Geometry check sheet. Reference: the model listing, model coordinates, mm. Coordinates: 2 decimals unless noted, no trailing zeros. Loops run counter-clockwise (first coordinate to the right, second up) from the corner with the lowest first, then second, coordinate; pieces in that order, holes last. Notation, with made-up numbers: (29, 58) - (46, 58) arc R14 cw to (46, 78) - close; hole circle Ø6 at (37.25, 18.25). An arc over 180 degrees is marked (long way). One line per item, written item: value.
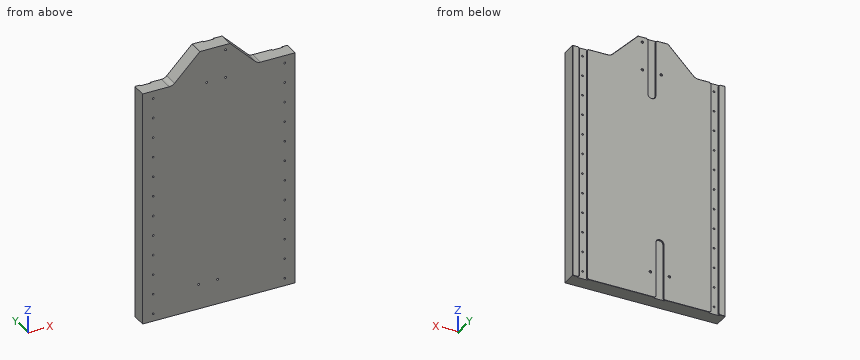
from build123d import *

# Parameters (mm, degrees)
BOSS_EXTRUDE1_DEPTH = 30
SKETCH2_R           = 1.75
SKETCH2_R_2         = 2
CUT_EXTRUDE1_DEPTH  = 31
SKETCH3_W           = 15.25
SKETCH3_H           = 470
CUT_EXTRUDE2_DEPTH  = 3
SKETCH4_W           = 15
SKETCH4_H           = 120
CUT_EXTRUDE3_DEPTH  = 3
FILLET1_R           = 7
FILLET2_R           = 15
CHAMFER1_SIZE       = 3
CHAMFER2_SIZE       = 0.5


with BuildPart() as part:
    # Sketch1 → Boss-Extrude1 (new body)
    with BuildSketch(Plane(origin=(0, 0, 0), x_dir=(1, 0, 0), z_dir=(0, 1, 0))):
        Polygon((-93, -235), (-38, -290), (22, -290), (77, -235), (152.5, -235), (152.5, 235), (-152.5, 235), (-152.5, -235), align=None)
    extrude(amount=BOSS_EXTRUDE1_DEPTH)

    # Sketch2 → Cut-Extrude1 (cut, through all)
    with BuildSketch(Plane(origin=(0, 0, 0), x_dir=(1, 0, 0), z_dir=(0, 1, 0))):
        with Locations((-131.5, 220)):
            Circle(SKETCH2_R)
        with Locations((131.5, 220)):
            Circle(SKETCH2_R)
        with Locations((13.5, -223)):
            Circle(SKETCH2_R_2)
        with Locations((-24.5, -223)):
            Circle(SKETCH2_R_2)
        with Locations((-40.5, 185)):
            Circle(SKETCH2_R_2)
        with Locations((-2.5, 185)):
            Circle(SKETCH2_R_2)
        with Locations((-131.5, 180)):
            Circle(SKETCH2_R)
        with Locations((131.5, 180)):
            Circle(SKETCH2_R)
        with Locations((-131.5, 140)):
            Circle(SKETCH2_R)
        with Locations((131.5, 140)):
            Circle(SKETCH2_R)
        with Locations((-131.5, 100)):
            Circle(SKETCH2_R)
        with Locations((131.5, 100)):
            Circle(SKETCH2_R)
        with Locations((-131.5, 60)):
            Circle(SKETCH2_R)
        with Locations((131.5, 60)):
            Circle(SKETCH2_R)
        with Locations((-131.5, 20)):
            Circle(SKETCH2_R)
        with Locations((131.5, 20)):
            Circle(SKETCH2_R)
        with Locations((-131.5, -20)):
            Circle(SKETCH2_R)
        with Locations((131.5, -20)):
            Circle(SKETCH2_R)
        with Locations((-131.5, -60)):
            Circle(SKETCH2_R)
        with Locations((131.5, -60)):
            Circle(SKETCH2_R)
        with Locations((-131.5, -100)):
            Circle(SKETCH2_R)
        with Locations((131.5, -100)):
            Circle(SKETCH2_R)
        with Locations((-131.5, -140)):
            Circle(SKETCH2_R)
        with Locations((131.5, -140)):
            Circle(SKETCH2_R)
        with Locations((-131.5, -180)):
            Circle(SKETCH2_R)
        with Locations((131.5, -180)):
            Circle(SKETCH2_R)
        with Locations((-131.5, -220)):
            Circle(SKETCH2_R)
        with Locations((131.5, -220)):
            Circle(SKETCH2_R)
        with Locations((13.5, -279.5)):
            Circle(SKETCH2_R_2)
    extrude(amount=CUT_EXTRUDE1_DEPTH, mode=Mode.SUBTRACT)

    # Sketch3 → Cut-Extrude2 (cut)
    with BuildSketch(Plane(origin=(0, 30, 0), x_dir=(1, 0, 0), z_dir=(0, 1, 0))):
        with Locations((-131.5, 0)):
            Rectangle(SKETCH3_W, SKETCH3_H)
        with Locations((131.5, 0)):
            Rectangle(SKETCH3_W, SKETCH3_H)
    extrude(amount=-CUT_EXTRUDE2_DEPTH, mode=Mode.SUBTRACT)

    # Sketch4 → Cut-Extrude3 (cut)
    with BuildSketch(Plane(origin=(0, 30, 0), x_dir=(1, 0, 0), z_dir=(0, 1, 0))):
        with Locations((-5.5, -230)):
            Rectangle(SKETCH4_W, SKETCH4_H)
        with Locations((-21.5, 175)):
            Rectangle(SKETCH4_W, SKETCH4_H)
    extrude(amount=-CUT_EXTRUDE3_DEPTH, mode=Mode.SUBTRACT)

    # Fillet1
    fillet1_edges = [part.edges().sort_by_distance(p)[0] for p in [
        (-13, 28.5, 170),
        (2, 28.5, 170),
        (-29, 28.5, -115),
        (-14, 28.5, -115),
    ]]
    fillet(fillet1_edges, radius=FILLET1_R)

    # Fillet2
    fillet2_edges = [part.edges().sort_by_distance(p)[0] for p in [
        (77, 15, 235),
        (-93, 15, 235),
    ]]
    fillet(fillet2_edges, radius=FILLET2_R)

    # Chamfer1
    chamfer1_edges = [part.edges().sort_by_distance(p)[0] for p in [
        (-123.875, 28.5, -235),
        (-123.875, 28.5, 235),
        (-139.125, 28.5, 235),
        (-139.125, 28.5, -235),
        (123.875, 28.5, 235),
        (123.875, 28.5, -235),
        (139.125, 28.5, -235),
        (139.125, 28.5, 235),
        (-13, 28.5, 290),
        (2, 28.5, 290),
        (-29, 28.5, -235),
        (-14, 28.5, -235),
    ]]
    chamfer(chamfer1_edges, length=CHAMFER1_SIZE)

    # Chamfer2
    chamfer2_edges = [part.edges().sort_by_distance(p)[0] for p in [
        (-152.5, 30, 0),
        (-147.3125, 30, 235),
        (-27, 30, 290),
        (47.303300859, 30, 264.696699141),
        (-21.5, 30, -115),
        (-14, 30, -177),
        (-13, 30, 232),
        (-5.5, 30, 170),
        (-26.949747468, 30, -117.050252532),
        (-16.050252532, 30, -117.050252532),
        (-10.949747468, 30, 172.050252532),
        (-0.050252532, 30, 172.050252532),
        (102.044101718, 30, 235),
        (-63.303300859, 30, 264.696699141),
        (77.47295195, 30, 236.141807012),
        (-93.47295195, 30, 236.141807012),
        (-110.044101718, 30, 235),
        (-139.125, 30, 0),
        (-147.3125, 30, -235),
        (-140.625, 30, -233.5),
        (-140.625, 30, 233.5),
        (-123.875, 30, 0),
        (2, 30, 232),
        (13.5, 30, 290),
        (123.875, 30, 0),
        (54.9375, 30, -235),
        (-29, 30, -177),
        (-76.4375, 30, -235),
        (-14.5, 30, 288.5),
        (3.5, 30, 288.5),
        (-30.5, 30, -233.5),
        (-12.5, 30, -233.5),
        (-122.375, 30, -233.5),
        (122.375, 30, -233.5),
        (122.375, 30, 233.5),
        (-122.375, 30, 233.5),
        (139.125, 30, 0),
        (147.3125, 30, 235),
        (140.625, 30, -233.5),
        (140.625, 30, 233.5),
        (152.5, 30, 0),
        (147.3125, 30, -235),
        (11.5, 30, 223),
        (-26.5, 30, 223),
        (-42.5, 30, -185),
        (-4.5, 30, -185),
        (11.5, 30, 279.5),
    ]]
    chamfer(chamfer2_edges, length=CHAMFER2_SIZE)


solid = part.part
(1) Cross-section at C-C on x = 91.5. Record the cut outline in (y, z).
Reply:
outline: (0, -235) - (29.5, -235) - (30, -234.5) - (30, 234.5) - (29.5, 235) - (0, 235) - close
(2) Go/stop test with flat-tipped pins: pin 1 Ø4.5 at (x, z) = (131.5, 220) entering from -Y; pin 2 Ø2 at (x, z) = (131.5, 60) entering from -Y; pin 3 Ø9 at (x, y) = (111, 11) entering from +Z; pin 4 Ø0.8 at (x, y) = (-21.5, 28) entering from -Z. Record where each tip stops, or that it passes through.
Reply:
pin 1: y = 0
pin 2: through
pin 3: z = 235
pin 4: z = -115
(3) Material ranges on probe 1 along X at (y, z) = (17, 60); probe 2 along X at (y, z) = (28.5, -73) (3 decimals); probe 3 along X at (y, z) = (28, 255.5), recorded low to high. Write a range as from..to.
Reply:
probe 1: -152.5..-133.25, -129.75..129.75, 133.25..152.5
probe 2: -152.5..-139.125, -123.875..123.875, 139.125..152.5
probe 3: -72.5..-13, 2..56.5
(4) Cross-section at A-A on z = -199. Record the cut outline in (x, y) (3 decimals), and give its area (3 significant figures).
Reply:
outline: (-152.5, 0) - (152.5, 0) - (152.5, 29.5) - (152, 30) - (139.625, 30) - (139.125, 29.5) - (139.125, 27) - (123.875, 27) - (123.875, 29.5) - (123.375, 30) - (-13.5, 30) - (-14, 29.5) - (-14, 27) - (-29, 27) - (-29, 29.5) - (-29.5, 30) - (-123.375, 30) - (-123.875, 29.5) - (-123.875, 27) - (-139.125, 27) - (-139.125, 29.5) - (-139.625, 30) - (-152, 30) - (-152.5, 29.5) - close
area: 9,010 mm2
(5) Cross-section at B-B on y = 14.5. State how many separate pieces and enclosed holes the cut face has, and give its area (3 significant figures).
Reply:
separate pieces: 1
enclosed holes: 29
area: 149,000 mm2
(6) Cross-section at D-D on x = -66. Record the cut outline in (y, z), and give its area (3 significant figures).
Reply:
outline: (0, -235) - (29.5, -235) - (30, -234.5) - (30, 261.29) - (29.5, 262) - (0, 262) - close
area: 14,900 mm2
